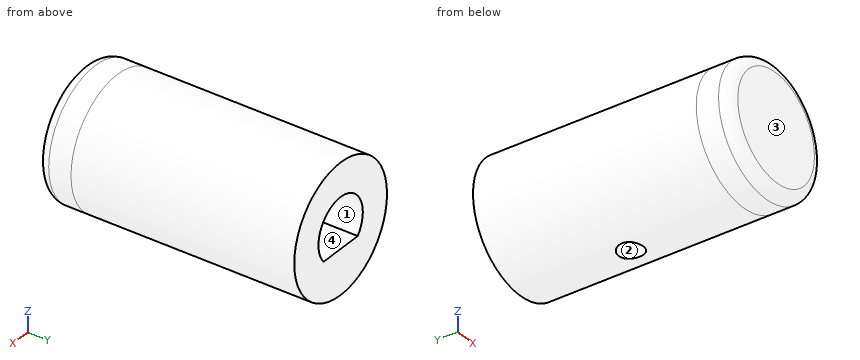
```python
from build123d import *

# Parameters (mm, degrees)
SKETCH1_R           = 5.75
SKETCH1_R_2         = 2.75
BOSS_EXTRUDE1_DEPTH = 20
BOSS_EXTRUDE3_START = -20
BOSS_EXTRUDE3_DEPTH = 20
SKETCH2_R           = 1.1
CUT_EXTRUDE1_DEPTH  = 22.589928207
BOSS_EXTRUDE2_START = 3
SKETCH3_R           = 5.75
BOSS_EXTRUDE2_DEPTH = 3
FILLET1_R           = 1


with BuildPart() as part:
    # Sketch1 → Boss-Extrude1 (new body)
    with BuildSketch(Plane(origin=(0, 0, 0), x_dir=(1, 0, 0), z_dir=(0, 1, 0))):
        with Locations(Location((0, 0, 0), (0, 0, 270))):
            Circle(SKETCH1_R)
        with Locations(Location((0, 0, 0), (0, 0, 270))):
            Circle(SKETCH1_R_2, mode=Mode.SUBTRACT)
    extrude(amount=BOSS_EXTRUDE1_DEPTH)

    # Sketch5 → Boss-Extrude3 (add)
    with BuildSketch(Plane(origin=(0, 20, 0), x_dir=(1, 0, 0), z_dir=(0, 1, 0)).offset(BOSS_EXTRUDE3_START)):
        with BuildLine():
            Line((-2.121320344, 1.75), (2.121320344, 1.75))
            ThreePointArc((2.121320344, 1.75), (0, 2.75), (-2.121320344, 1.75))
        make_face()
    extrude(amount=BOSS_EXTRUDE3_DEPTH)

    # Sketch2 → Cut-Extrude1 (cut, through all)
    with BuildSketch(Plane.XY):
        with Locations((0, 10)):
            Circle(SKETCH2_R)
    extrude(amount=-CUT_EXTRUDE1_DEPTH, mode=Mode.SUBTRACT)

    # Sketch3 → Boss-Extrude2 (add)
    with BuildSketch(Plane.XZ.offset(BOSS_EXTRUDE2_START)):
        with Locations(Location((0, 0, 0), (0, 0, 270))):
            Circle(SKETCH3_R)
    extrude(amount=-BOSS_EXTRUDE2_DEPTH)

    # Fillet1
    fillet1_edges = [part.edges().sort_by_distance(p)[0] for p in [
        (0, -3, 5.75),
    ]]
    fillet(fillet1_edges, radius=FILLET1_R)


solid = part.part
```
The model under review builds one solid part; all positions refer to its coordinate system, in mm. Face numbers are marked on the shaded views. A direction names the side the tool comes from. Give positions to 0.01 mm unless a question says otherwise; leave off trailing zeros. Write each loop counter-clockwise with the first axis right and the second up, starting at its lowest first coordinate (ties: lowest second). Pieces come first, ordered by that corner, then holes. Notation, with made-up numbers: (21, 9) -> (55, 9) arc R23 cw to (55, 33) -> close; hole circle Ø9 at (-17, 77). An arc over 180 degrees is marked (long way). Answer in a Markdown table with one row per item.
1) Tool access review of the marked faces 3 and 4: name each direction out of +Z, -Z, +X, -X, +Y, -Y from which nothing blocks a thin tool from reaching the whole face with its end or side.
Worked answers:
| item | result |
|---|---|
| face 3 | +Z, -Z, +X, -X, -Y |
| face 4 | +Y |
2) Add section D-D on y = 10.25. State the section outline as (x, z) points, plus the area to 3 significant figures.
Worked answers:
| item | result |
|---|---|
| outline | (-2.12, -1.75) arc R2.75 cw (long way) to (2.12, -1.75) -> (1.07, -1.75) -> (1.07, -5.65) arc R5.75 ccw (long way) to (-1.07, -5.65) -> (-1.07, -1.75) -> close |
| area | 74.6 mm² |
3) Add section C-C on y = 16.5. State the section outline as (x, z) points, plus the area to 3 significant figures.
Worked answers:
| item | result |
|---|---|
| outline | circle Ø11.5 at (0, 0); hole (-2.12, -1.75) -> (2.12, -1.75) arc R2.75 ccw (long way) to start |
| area | 83.1 mm² |
4) For L1, parallel to X at y = 12.75, z = 0; L2, parallel to Z at x = 0, y = 12.75; L3, parallel to Y at x = 0, z = -3.5, list the stretches that pass through material, from the lowest coordinate up. Write a range as [from, to].
Worked answers:
| item | result |
|---|---|
| L1 | [-5.75, -2.75], [2.75, 5.75] |
| L2 | [-5.75, -1.75], [2.75, 5.75] |
| L3 | [-3, 8.9], [11.1, 20] |
5) Add section A-A on x = 0. State the section outline as (y, z) points, plus the area to 3 significant figures.
Worked answers:
| item | result |
|---|---|
| outline | (-3, -4.75) arc R1 ccw to (-2, -5.75) -> (8.9, -5.75) -> (8.9, -1.75) -> (0, -1.75) -> (0, 2.75) -> (20, 2.75) -> (20, 5.75) -> (-2, 5.75) arc R1 ccw to (-3, 4.75) -> close; (11.1, -5.75) -> (20, -5.75) -> (20, -1.75) -> (11.1, -1.75) -> close |
| area | 165 mm² |
6) Clearance check with flat-ended pins moving along their axes: P1, Ø1, axis at x = 0, z = -1, coming from the +Y side; P2, Ø2, axis at y = 3, z = 2, coming from the -X side; P3, Ø1.5, axis at x = 1.5, y = 10, coming from the +Z side. State where each tip first meets the part, or that it passes through.
Worked answers:
| item | result |
|---|---|
| P1 | y = 0 |
| P2 | x = -5.66 |
| P3 | z = 5.7 |
7) Mouldability with a two-part tool opening along Z and no side actions: class the marked faces 1 and 2 as +Z half, -Z half, draft (parallel to the pull), parting line (faces both ways), or undercut.
Worked answers:
| item | result |
|---|---|
| face 1 | undercut |
| face 2 | draft |
8) Add section B-B on z = 0. State the section outline as (x, y) points, plus the area to 3 significant figures.
Worked answers:
| item | result |
|---|---|
| outline | (-5.75, -2) arc R1 ccw to (-4.75, -3) -> (4.75, -3) arc R1 ccw to (5.75, -2) -> (5.75, 20) -> (2.75, 20) -> (2.75, 0) -> (-2.75, 0) -> (-2.75, 20) -> (-5.75, 20) -> close |
| area | 154 mm² |
